Study the drawing (mm; zero at the part's minimum x, y, z) and answer. Coordinates: 2 decimals unless noted, no trailing zeros. Order: outer loops, then holes, each group sorted by start corner. A loop starts at its lowest first (then second) coordinate and runs counter-clockwise, first axis right, second up. Notation, with made-up numbers: M -6.75,11 L 9.25,11 A24 cw 9.25,24 Z; hole C 78.5,53 d4. An arc over 180 degrees is marked long. Use a Markdown table: item, result. Add a question column.
1) Find section B-B on z = 70. Write down the section's boundary in (x, y), plus the area to 3 significant figures.
2) Find section D-D on z = 43.5. Write down the section's boundary in (x, y).
3) The mould has two halves that part along Z. Classify the marked faces 1, 2 and 3: released by +Z, released by -Z, zero draft, split by the parting line, or undercut.
4) Find the intervals of material crossed by probe 1 along X at (y, z) = (1.55, 70); probe 2 along X at (y, z) = (10.5, 58) (1 decimal); probe 3 along Z at (x, y) = (85, 15) (1 decimal), in increasing order. Write a range as [from, to].
5) Find section C-C on y = 11. Write down the section's boundary in (x, z), plus the area to 3 significant figures.
6) Each of these flat-tipped pins is pushed along its axis until it touches: pin 1 Ø1.5 at (y, z) = (7.5, 97.5) entering from +X; pin 2 Ø9.5 at (x, z) = (75, 76.5) entering from +Y; pin 3 Ø3 at (x, y) = (36, 14.5) entering from -Z. Where does it stop, or does it pass through?
7) Find section A-A on x = 70. Write down the section's boundary in (y, z).
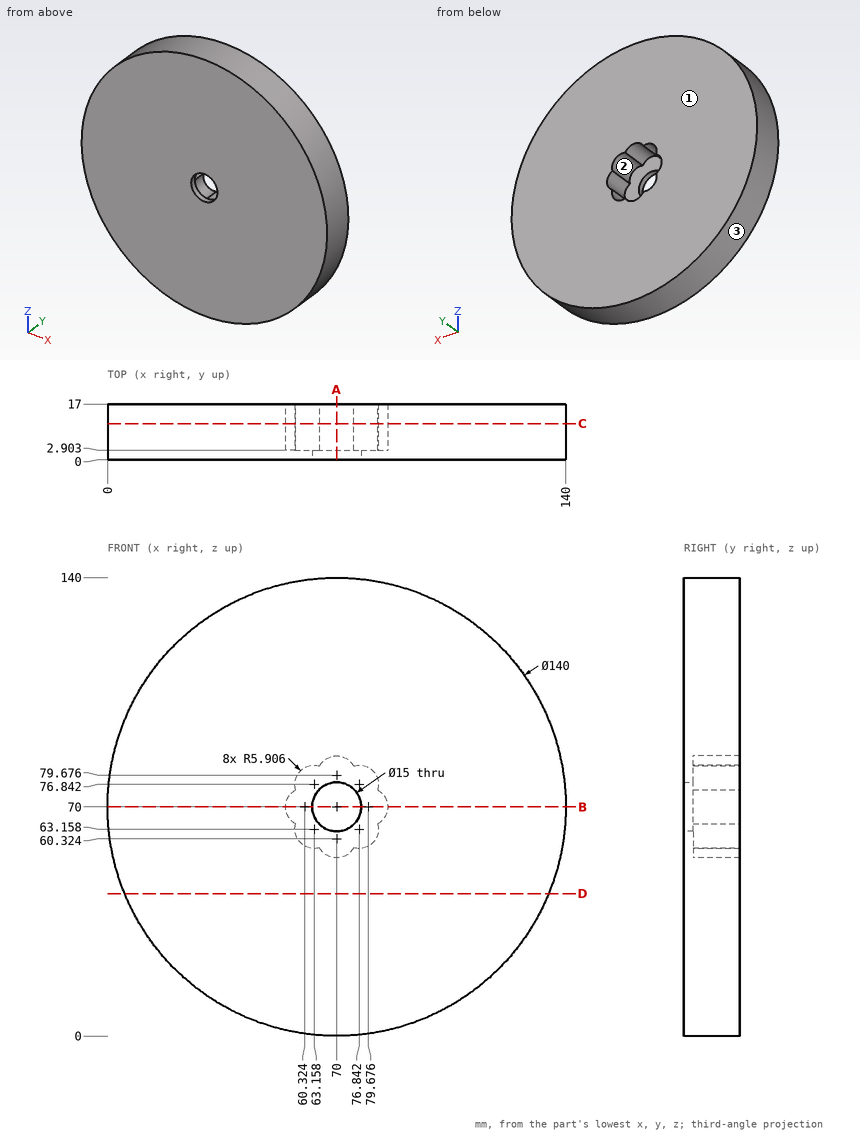
Check result:
| question | item | result |
|---|---|---|
| 1 | outline | M 0,0 L 62.5,0 L 62.5,2.9 L 54.42,2.9 L 54.42,17 L 0,17 Z; M 77.5,0 L 140,0 L 140,17 L 85.58,17 L 85.58,2.9 L 77.5,2.9 Z |
| 1 | area | 1,900 mm2 |
| 2 | outline | M 5.21,0 L 134.79,0 L 134.79,17 L 5.21,17 Z |
| 3 | face 1 | zero draft |
| 3 | face 2 | undercut |
| 3 | face 3 | split by the parting line |
| 4 | probe 1 | x = [0, 62.5], [77.5, 140] |
| 4 | probe 2 | x = [1, 60.3], [79.7, 139] |
| 4 | probe 3 | z = [1.6, 67.4], [72.6, 138.4] |
| 5 | outline | C 70,70 d140; hole M 57.49,64.82 A5.91 ccw 64.82,57.49 A5.91 ccw 75.18,57.49 A5.91 ccw 82.51,64.82 A5.91 ccw 82.51,75.18 A5.91 ccw 75.18,82.51 A5.91 ccw 64.82,82.51 A5.91 ccw 57.49,75.18 A5.91 ccw Z |
| 5 | area | 14,700 mm2 |
| 6 | pin 1 | stops at x = 134.69 |
| 6 | pin 2 | stops at y = 2.9 |
| 6 | pin 3 | stops at z = 8 |
| 7 | outline | M 0,0 L 17,0 L 17,54.42 L 2.9,54.42 L 2.9,62.5 L 0,62.5 Z; M 0,77.5 L 2.9,77.5 L 2.9,85.58 L 17,85.58 L 17,140 L 0,140 Z |
